```python
from build123d import *

# Parameters (mm, degrees)
SKETCH1_R               = 15
BOSS_EXTRUDE1_DEPTH     = 3.5
SKETCH3_R               = 13
BOSS_EXTRUDE2_DEPTH     = 1.5
SKETCH4_R               = 15
BOSS_EXTRUDE3_DEPTH     = 12
SKETCH5_R               = 13
BOSS_EXTRUDE4_DEPTH     = 1.5
SKETCH6_R               = 15
BOSS_EXTRUDE5_DEPTH     = 12
SKETCH7_R               = 13
BOSS_EXTRUDE6_DEPTH     = 1.5
SKETCH8_R               = 15
BOSS_EXTRUDE7_DEPTH     = 2.75
CUT_EXTRUDE1_DEPTH      = 41.713173544
CUT_EXTRUDE1_DEPTH_BACK = 41.713173544
SKETCH9_R               = 9
SKETCH12_R              = 9
BOSS_EXTRUDE9_DEPTH     = 2
CUT_EXTRUDE3_DEPTH      = 37.538507085
CUT_EXTRUDE3_DEPTH_BACK = 37.538507085
SKETCH13_R              = 1.5
SKETCH14_W              = 5
SKETCH14_H              = 34.75
BOSS_EXTRUDE10_DEPTH    = 1
CUT_EXTRUDE4_DEPTH      = 41.713173544
CUT_EXTRUDE4_DEPTH_BACK = 41.713173544
SKETCH15_R              = 15.408664216
SKETCH15_R_2            = 15


with BuildPart() as part:
    # Sketch1 → Boss-Extrude1 (new body)
    with BuildSketch(Plane(origin=(0, 0, 0), x_dir=(1, 0, 0), z_dir=(0, 1, 0))):
        with Locations(Location((0, 0, 0), (0, 0, 270))):
            Circle(SKETCH1_R)
    extrude(amount=BOSS_EXTRUDE1_DEPTH)

    # Sketch3 → Boss-Extrude2 (add)
    with BuildSketch(Plane(origin=(0, 3.5, 0), x_dir=(1, 0, 0), z_dir=(0, 1, 0))):
        with Locations(Location((0, 0, 0), (0, 0, 270))):
            Circle(SKETCH3_R)
    extrude(amount=BOSS_EXTRUDE2_DEPTH)

    # Sketch4 → Boss-Extrude3 (add)
    with BuildSketch(Plane(origin=(0, 5, 0), x_dir=(1, 0, 0), z_dir=(0, 1, 0))):
        with Locations(Location((0, 0, 0), (0, 0, 270))):
            Circle(SKETCH4_R)
    extrude(amount=BOSS_EXTRUDE3_DEPTH)

    # Sketch5 → Boss-Extrude4 (add)
    with BuildSketch(Plane(origin=(0, 17, 0), x_dir=(1, 0, 0), z_dir=(0, 1, 0))):
        with Locations(Location((0, 0, 0), (0, 0, 270))):
            Circle(SKETCH5_R)
    extrude(amount=BOSS_EXTRUDE4_DEPTH)

    # Sketch6 → Boss-Extrude5 (add)
    with BuildSketch(Plane(origin=(0, 18.5, 0), x_dir=(1, 0, 0), z_dir=(0, 1, 0))):
        with Locations(Location((0, 0, 0), (0, 0, 270))):
            Circle(SKETCH6_R)
    extrude(amount=BOSS_EXTRUDE5_DEPTH)

    # Sketch7 → Boss-Extrude6 (add)
    with BuildSketch(Plane(origin=(0, 30.5, 0), x_dir=(1, 0, 0), z_dir=(0, 1, 0))):
        with Locations(Location((0, 0, 0), (0, 0, 270))):
            Circle(SKETCH7_R)
    extrude(amount=BOSS_EXTRUDE6_DEPTH)

    # Sketch8 → Boss-Extrude7 (add)
    with BuildSketch(Plane(origin=(0, 32, 0), x_dir=(1, 0, 0), z_dir=(0, 1, 0))):
        with Locations(Location((0, 0, 0), (0, 0, 270))):
            Circle(SKETCH8_R)
    extrude(amount=BOSS_EXTRUDE7_DEPTH)

    # Sketch9 → Cut-Extrude1 (cut, two sides: drawn at the far end of the back side and taken through both)
    with BuildSketch(Plane(origin=(0, 0, 0), x_dir=(1, 0, 0), z_dir=(0, 1, 0)).offset(-CUT_EXTRUDE1_DEPTH_BACK)):
        with Locations(Location((0, 0, 0), (0, 0, 270))):
            Circle(SKETCH9_R)
    extrude(amount=CUT_EXTRUDE1_DEPTH + CUT_EXTRUDE1_DEPTH_BACK, mode=Mode.SUBTRACT)

    # Sketch12 → Boss-Extrude9 (add)
    with BuildSketch(Plane(origin=(0, 5, 0), x_dir=(1, 0, 0), z_dir=(0, 1, 0))):
        with Locations(Location((0, 0, 0), (0, 0, 270))):
            Circle(SKETCH12_R)
    extrude(amount=BOSS_EXTRUDE9_DEPTH)

    # Sketch13 → Cut-Extrude3 (cut, two sides: drawn at the far end of the back side and taken through both)
    with BuildSketch(Plane(origin=(0, 5, 0), x_dir=(1, 0, 0), z_dir=(0, 1, 0)).offset(-CUT_EXTRUDE3_DEPTH_BACK)):
        with Locations(Location((0, 0, 0), (0, 0, 270))):
            Circle(SKETCH13_R)
        with Locations(Location((0, 7, 0), (0, 0, 270))):
            Circle(SKETCH13_R)
        with Locations(Location((0, -7, 0), (0, 0, 270))):
            Circle(SKETCH13_R)
        with Locations(Location((7, 0, 0), (0, 0, 270))):
            Circle(SKETCH13_R)
        with Locations(Location((-7, 0, 0), (0, 0, 270))):
            Circle(SKETCH13_R)
    extrude(amount=CUT_EXTRUDE3_DEPTH + CUT_EXTRUDE3_DEPTH_BACK, mode=Mode.SUBTRACT)

    # Sketch14 → Boss-Extrude10 (add)
    with BuildSketch(Plane(origin=(-15, 0, 0), x_dir=(0, 0, -1), z_dir=(1, 0, 0))):
        with Locations((0, 17.375)):
            Rectangle(SKETCH14_W, SKETCH14_H)
    extrude(amount=BOSS_EXTRUDE10_DEPTH)

    # Sketch15 → Cut-Extrude4 (cut, two sides: drawn at the far end of the back side and taken through both)
    with BuildSketch(Plane(origin=(0, 34.75, 0), x_dir=(1, 0, 0), z_dir=(0, 1, 0)).offset(-CUT_EXTRUDE4_DEPTH_BACK)):
        Circle(SKETCH15_R)
        with Locations(Location((0, 0, 0), (0, 0, 270))):
            Circle(SKETCH15_R_2, mode=Mode.SUBTRACT)
    extrude(amount=CUT_EXTRUDE4_DEPTH + CUT_EXTRUDE4_DEPTH_BACK, mode=Mode.SUBTRACT)


solid = part.part
```
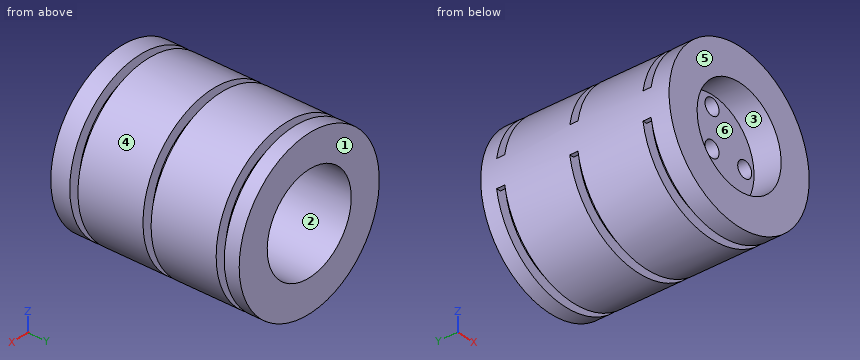
Check sheet for the modelled part. Datum: model origin and axes. Units: mm. Face numbers are marked on the shaded views. A direction names the side the tool comes from. Give positions to 0.01 mm unless a question says otherwise; leave off trailing zeros. Write each loop counter-clockwise with the first axis right and the second up, starting at its lowest first coordinate (ties: lowest second). Pieces come first, ordered by that corner, then holes. Notation, with made-up numbers: (19, 68.25) - (60, 68.25) arc R24 ccw to (60, 97.25) - close; hole circle Ø10 at (44, 21.25). An arc over 180 degrees is marked (long way). Answer as a JSON object with one key per item and string values. Group by question number.
1) Thickness scan on probe 1 along Y at (x, z) = (-12.5, -5.5); probe 2 along X at (y, z) = (5.8, 0). Record the ranges inside material, lowest first. Write a range as from..to.
2) Release check for a two-part mould opening along X. For the marked faces 1, 2, 3 and 4 record: pulls with the +X half, pulls with the -X half, needs draft (parallel to the pull), parting line crosses it, or undercut.
3) Access from +Z, -Z, +X, -X, +Y, -Y to the whole of each face (thin tool, end or side, straight path). Record for the marked faces 5 and 6.
4) Sectioned sample at A-A (x = 10). Record the cut outline in (y, z).
5) Sectioned sample at B-B (y = 26). Record the cut outline in (x, z), then the cut area to 3 significant figures.
6) Depth check by flat-ended pin: P1, Ø8, axis at x = -8.5, z = 7, coming from the -Y side; P2, Ø0.9, axis at x = -14.5, y = 31.5, coming from the -Z side; P3, Ø12, axis at x = -9, y = 12, coming from the -Z side; P4, Ø5, axis at y = 6, z = -5.5, coming from the +X side. Enter the tip coordinate at first touch or a pass-through.
Geometry results:
{
 "1": {"probe 1": "y = 0..3.5, 5..17, 18.5..30.5, 32..34.75", "probe 2": "x = -15..-8.5, -5.5..-1.5, 1.5..5.5, 8.5..15"},
 "2": {"face 1": "needs draft", "face 2": "undercut", "face 3": "undercut", "face 4": "parting line crosses it"},
 "3": {"face 5": "+Z, -Z, +X, -X, -Y", "face 6": "-Y"},
 "4": {"outline": "(0, -11.18) - (3.5, -11.18) - (3.5, -8.31) - (5, -8.31) - (5, -11.18) - (17, -11.18) - (17, -8.31) - (18.5, -8.31) - (18.5, -11.18) - (30.5, -11.18) - (30.5, -8.31) - (32, -8.31) - (32, -11.18) - (34.75, -11.18) - (34.75, 11.18) - (32, 11.18) - (32, 8.31) - (30.5, 8.31) - (30.5, 11.18) - (18.5, 11.18) - (18.5, 8.31) - (17, 8.31) - (17, 11.18) - (5, 11.18) - (5, 8.31) - (3.5, 8.31) - (3.5, 11.18) - (0, 11.18) - close"},
 "5": {"outline": "circle Ø30 at (0, 0); hole circle Ø18 at (0, 0)", "area": "452 mm^2"},
 "6": {"P1": "stops at y = 0", "P2": "stops at z = -2.5", "P3": "stops at z = -14.7", "P4": "stops at x = 14.7"}
}
